from build123d import *

# Parameters (mm, degrees)
BOSS_EXTRUDE1_DEPTH          = 6.35
F_10_0_1935_DIAMETER_HOLE1_D = 4.9149


with BuildPart() as part:
    # Sketch1 → Boss-Extrude1 (new body)
    with BuildSketch(Plane(origin=(0, 0, 0), x_dir=(1, 0, 0), z_dir=(0, 1, 0))):
        Polygon((0, 60.325), (-9.525, 37.329615818), (-9.525, -37.329615818), (0, -60.325), (9.525, -37.329615818), (9.525, 37.329615818), align=None)
    extrude(amount=BOSS_EXTRUDE1_DEPTH)

    # #10 (0.1935) Diameter Hole1 (through all)
    with Locations(Plane(origin=(0, 6.35, 0), x_dir=(1, 0, 0), z_dir=(0, 1, 0))):
        with Locations((0, 20.32), (0, 40.64), (0, 0), (0, -20.32), (0, -40.64)):
            Hole(F_10_0_1935_DIAMETER_HOLE1_D / 2)


solid = part.part
Could you check a few things on this model? Use its own coordinates, in mm. Give positions to 0.01 mm unless a question says otherwise; leave off trailing zeros. Order: outer loops, then holes, each group sorted by start corner. A loop starts at its lowest first (then second) coordinate and runs counter-clockwise, first axis right, second up.
Item 1: I'm going to push flat-ended pins straight in: pin 1 (3 mm diameter, centred on x = -7.5, y = 5.5, fed in from +Z); pin 2 (1.5 mm diameter, centred on x = -2.5, y = 4, fed in from +Z). Where does each tip first touch, or does it pass through?
Item 2: If we section it at C-C, the plane x = -6.75: Write out the boundary of the cut face in (y, z), plus the area to 3 significant figures.
Item 3: If we section it at B-B, the plane y = 5: Write out the boundary of the cut face in (x, z) (3 decimals), plus the area to 3 significant figures.
Item 4: If we section it at A-A, the plane z = 0: Write out the boundary of the cut face in (x, y) (3 decimals), plus the area to 3 significant figures.
Item 5: I need wall thicknesses on line 1 (X direction, y = 2, z = 20.32) (3 decimals); line 2 (Z direction, x = 1, y = 3.25); line 3 (Z direction, x = -1.5, y = 5.5). Which ranges of each line are inside material? Lowest first, please.
Item 6: If we mould it in two halves opening along Z, with no side actions, what happens to faces 1 (the face through (-1.321, 3.131, 38.568)), 2 (the face through (4.829, 3.131, -48.666)), 3 (the face through (-4, 6.35, -1)), 4 (the face through (-1.321, 3.131, -42.712))? For each: pulls with the +Z half, pulls with the -Z half, needs draft (parallel to the pull), parting line crosses it, or undercut.
Values:
1. pin 1: stops at z = 45.84
1. pin 2: stops at z = 56.1
2. outline: (0, -44.03) - (6.35, -44.03) - (6.35, 44.03) - (0, 44.03) - close
2. area: 559 mm2
3. outline: (-9.525, -37.33) - (0, -60.325) - (9.525, -37.33) - (9.525, 37.33) - (0, 60.325) - (-9.525, 37.33) - close; hole circle Ø4.915 at (0, -40.64); hole circle Ø4.915 at (0, -20.32); hole circle Ø4.915 at (0, 0); hole circle Ø4.915 at (0, 20.32); hole circle Ø4.915 at (0, 40.64)
3. area: 1,770 mm2
4. outline: (-9.525, 0) - (-2.457, 0) - (-2.457, 6.35) - (-9.525, 6.35) - close; (2.457, 0) - (9.525, 0) - (9.525, 6.35) - (2.457, 6.35) - close
4. area: 89.8 mm2
5. line 1: x = -9.525 to -2.457, 2.457 to 9.525
5. line 2: z = -57.91 to -42.88, -38.4 to -22.56, -18.08 to -2.24, 2.24 to 18.08, 22.56 to 38.4, 42.88 to 57.91
5. line 3: z = -56.7 to -42.59, -38.69 to -22.27, -18.37 to -1.95, 1.95 to 18.37, 22.27 to 38.69, 42.59 to 56.7
6. face 1: undercut
6. face 2: pulls with the -Z half
6. face 3: needs draft
6. face 4: undercut
